The model under review builds one solid part; all positions refer to its coordinate system, in mm. Face numbers are marked on the shaded views. A direction names the side the tool comes from. Coordinates: 2 decimals unless noted, no trailing zeros. Order: outer loops, then holes, each group sorted by start corner. A loop starts at its lowest first (then second) coordinate and runs counter-clockwise, first axis right, second up. Notation, with made-up numbers: M 27,-13 L 35,-13 A24 ccw 35,7 Z; hole C 73,69 d2. An arc over 180 degrees is marked long. Answer as CSV lines item,"result". Start each with the question number.
Q1. Machinability: for the marked faces 4 and 5, which of the approach directions +Z, -Z, +X, -X, +Y, -Y give a long, thin tool a straight path to every point of the face, cutting with its end or side? Answer none if there is none.
Q2. Consider section A-A on x = 0. Write out the cut boundary in (y, z), and give its area (3 significant figures).
Q3. Consider section C-C on y = 3.2. State how many separate pieces and enclosed holes the cut face has, and give its area (3 significant figures).
Q4. Wall thickness on L1, parallel to Z at x = 5, y = 0.45; L2, parallel to X at y = 0.3, z = 4.5; L3, parallel to X at y = 3.95, z = -2.5: over which ranges is each line inside the solid? List them lowest first. Write a range as [from, to].
Q5. Consider section B-B on z = -11.5. Write out the cut boundary in (x, y), and give its area (3 significant figures).
Q6. Consider section D-D on x = -8.5. Write out the cut boundary in (y, z), and give its area (3 significant figures).
Q7. The part is to be moulded in two halves that separate along X. For the marked faces 1, 2 and 3, say which applies: +X half, -X half, draft (parallel to the pull), parting line (faces both ways), or undercut.
Q8. For P1, Ø3, axis at x = -9.06, z = -17.27, coming from the +Y side; P2, Ø19, axis at x = 0, z = 0, coming from the -Y side; P3, Ø1.5, axis at y = 3, z = -17, coming from the +X side; P4, Ø3, axis at y = 2.5, z = -9, coming from the +X side, all flat-tipped, find the tip position at first contact; note any pin that passes through.
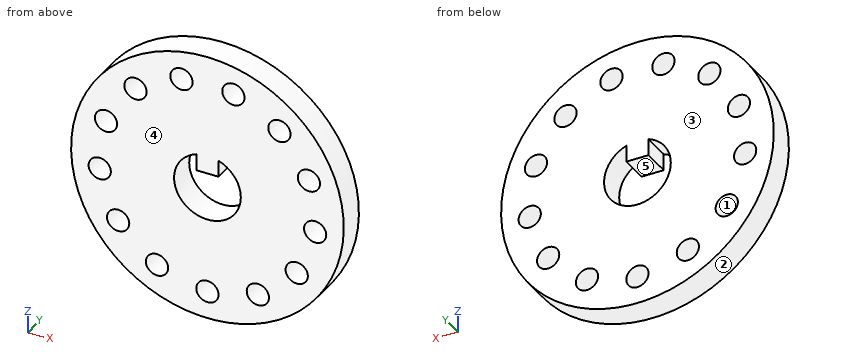
from build123d import *

# Parameters (mm, degrees)
SKETCH1_R           = 24.5
SKETCH1_R_2         = 2
BOSS_EXTRUDE1_DEPTH = 5


with BuildPart() as part:
    # Sketch1 → Boss-Extrude1 (new body)
    with BuildSketch(Plane(origin=(0, 0, 0), x_dir=(1, 0, 0), z_dir=(0, 1, 0))):
        with Locations(Location((0, 0, 0), (0, 0, 270))):
            Circle(SKETCH1_R)
        with Locations(Location((0, 19.5, 0), (0, 0, 270))):
            Circle(SKETCH1_R_2, mode=Mode.SUBTRACT)
        with Locations(Location((9.062101855, 17.2663925, 0), (0, 0, 270))):
            Circle(SKETCH1_R_2, mode=Mode.SUBTRACT)
        with Locations(Location((16.048185385, 11.077262561, 0), (0, 0, 270))):
            Circle(SKETCH1_R_2, mode=Mode.SUBTRACT)
        with Locations(Location((19.357823045, 2.350465265, 0), (0, 0, 270))):
            Circle(SKETCH1_R_2, mode=Mode.SUBTRACT)
        with Locations(Location((18.232816732, -6.914795297, 0), (0, 0, 270))):
            Circle(SKETCH1_R_2, mode=Mode.SUBTRACT)
        with Locations(Location((12.930891836, -14.595959589, 0), (0, 0, 270))):
            Circle(SKETCH1_R_2, mode=Mode.SUBTRACT)
        with Locations(Location((4.666655454, -18.93336544, 0), (0, 0, 270))):
            Circle(SKETCH1_R_2, mode=Mode.SUBTRACT)
        with Locations(Location((-4.666655454, -18.93336544, 0), (0, 0, 270))):
            Circle(SKETCH1_R_2, mode=Mode.SUBTRACT)
        with Locations(Location((-12.930891836, -14.595959589, 0), (0, 0, 270))):
            Circle(SKETCH1_R_2, mode=Mode.SUBTRACT)
        with Locations(Location((-18.232816732, -6.914795297, 0), (0, 0, 270))):
            Circle(SKETCH1_R_2, mode=Mode.SUBTRACT)
        with Locations(Location((-19.357823045, 2.350465265, 0), (0, 0, 270))):
            Circle(SKETCH1_R_2, mode=Mode.SUBTRACT)
        with Locations(Location((-16.048185385, 11.077262561, 0), (0, 0, 270))):
            Circle(SKETCH1_R_2, mode=Mode.SUBTRACT)
        with Locations(Location((-9.062101855, 17.2663925, 0), (0, 0, 270))):
            Circle(SKETCH1_R_2, mode=Mode.SUBTRACT)
        with BuildLine():
            Line((2, -5.656854249), (2, -2.656854249))
            Line((2, -2.656854249), (-2, -2.656854249))
            Line((-2, -2.656854249), (-2, -5.656854249))
            ThreePointArc((-2, -5.656854249), (0, 6), (2, -5.656854249))
        make_face(mode=Mode.SUBTRACT)
    extrude(amount=BOSS_EXTRUDE1_DEPTH)


solid = part.part
Evaluation:
1,face 4,"+Z, -Z, +X, -X, -Y"
1,face 5,"+Y, -Y"
2,outline,"M 0,-24.5 L 5,-24.5 L 5,-21.5 L 0,-21.5 Z; M 0,-17.5 L 5,-17.5 L 5,-6 L 0,-6 Z; M 0,2.66 L 5,2.66 L 5,24.5 L 0,24.5 Z"
2,area,"182 mm²"
3,separate pieces,"1"
3,enclosed holes,"14"
3,area,"1,620 mm²"
4,L1,"z = [-23.98, -3.32], [3.32, 16.96], [20.91, 23.98]"
4,L2,"x = [-24.08, -3.97], [-2, 2], [3.97, 24.08]"
4,L3,"x = [-24.37, -21.35], [-17.36, -5.45], [5.45, 17.36], [21.35, 24.37]"
5,outline,"M -21.63,0 L -18,0 L -18,5 L -21.63,5 Z; M -14.09,0 L 14.09,0 L 14.09,5 L -14.09,5 Z; M 18,0 L 21.63,0 L 21.63,5 L 18,5 Z"
5,area,"177 mm²"
6,outline,"M 0,-22.98 L 5,-22.98 L 5,-19.19 L 0,-19.19 Z; M 0,-15.35 L 5,-15.35 L 5,22.98 L 0,22.98 Z"
6,area,"211 mm²"
7,face 1,"undercut"
7,face 2,"parting line"
7,face 3,"draft"
8,P1,"passes through"
8,P2,"stops at y = 0"
8,P3,"stops at x = 18.34"
8,P4,"stops at x = 23.32"
